Job drawing, mm, ordinate dimensions from the low corner. One solid piece. A direction names the side the tool comes from. Round coordinates to 2 decimals unless told otherwise and drop trailing zeros. Loops run counter-clockwise (first coordinate to the right, second up) from the corner with the lowest first, then second, coordinate; pieces in that order, holes last.
1) Band-saw the part on A-A, the plane y = 3. Write the cut outline in (x, z), then the cut area to 3 significant figures.
2) Band-saw the part on B-B, the plane x = 3. Write the cut outline in (y, z).
3) Band-saw the part on C-C, the plane z = 17. Write the cut outline in (x, y).
4) Band-saw the part on D-D, the plane x = 7. Write the cut outline in (y, z).
5) Probe line 1 (Z direction, x = 35.5, y = 20.75); line 2 (X direction, y = 4.75, z = 17); line 3 (Y direction, x = 26, z = 21.5). List the from-to ranges inside material, lowest first.
6) 3-axis set-ups, long thin cutter, end or side, ignore diameter. For the marked faces 1, 2 and 3: which of +Z, -Z, +X, -X, +Y, -Y reach the whole face in a straight line?
7) Drop flat-ended pins along their axis: P1, Ø2, axis at x = 29.5, z = 14.5, coming from the -Y side; P2, Ø7, axis at x = 32.5, y = 2.5, coming from the +Z side; P3, Ø1, axis at x = 22.5, z = 15.5, coming from the -Y side. Give the stop position or say it passes through.
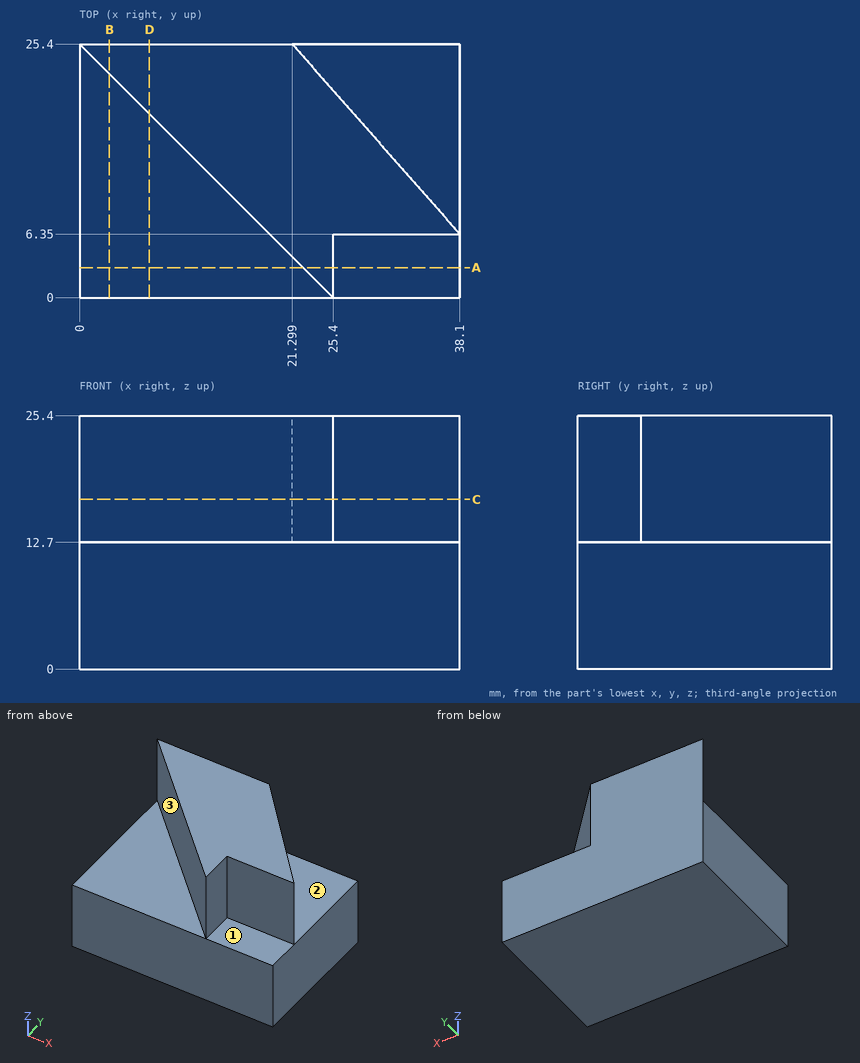
Reported:
1. outline: (0, 0) - (38.1, 0) - (38.1, 12.7) - (25.4, 12.7) - (25.4, 25.4) - (22.4, 25.4) - (22.4, 12.7) - (0, 12.7) - close
1. area: 522 mm2
2. outline: (0, 0) - (25.4, 0) - (25.4, 25.4) - (22.4, 25.4) - (22.4, 12.7) - (0, 12.7) - close
3. outline: (0, 25.4) - (25.4, 0) - (25.4, 6.35) - (38.1, 6.35) - (21.3, 25.4) - close
4. outline: (0, 0) - (25.4, 0) - (25.4, 25.4) - (18.4, 25.4) - (18.4, 12.7) - (0, 12.7) - close
5. line 1: z = 0 to 12.7
5. line 2: x = 20.65 to 25.4
5. line 3: y = 6.35 to 20.07
6. face 1: +Z, +X, -Y
6. face 2: +Z, +X, +Y
6. face 3: +Z, -X, -Y
7. P1: stops at y = 6.35
7. P2: stops at z = 12.7
7. P3: stops at y = 2.4
